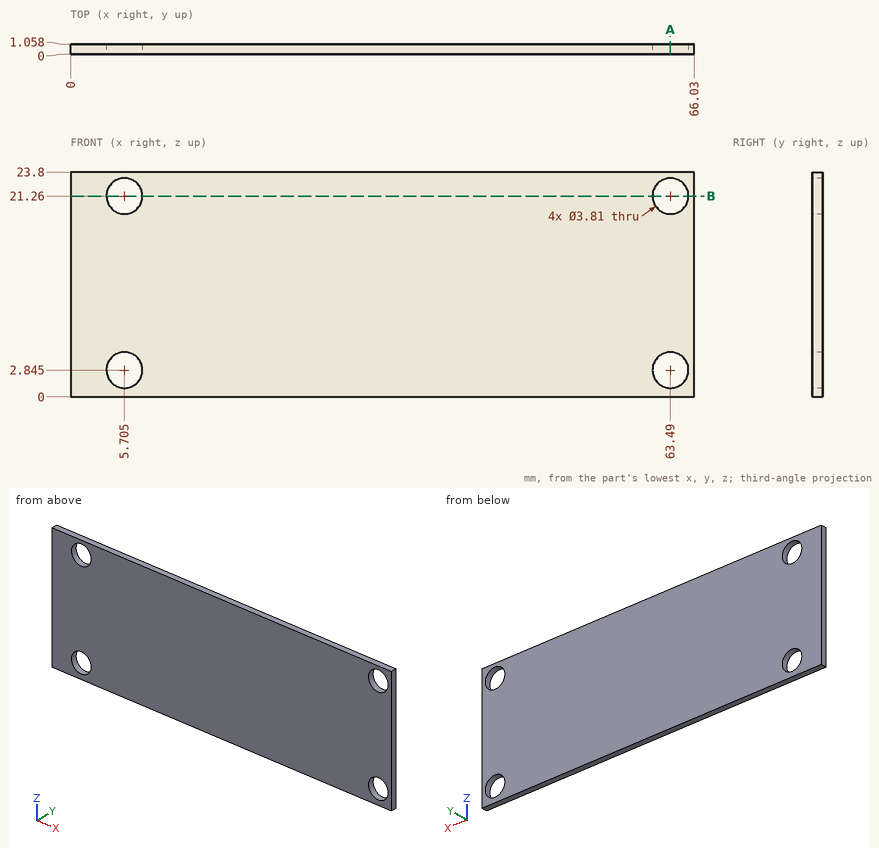
Source: three-view drawing plus pictorial views. Frame: mm from the lowest corner of the part. Coordinates: 2 decimals unless noted, no trailing zeros. Order: outer loops, then holes, each group sorted by start corner. A loop starts at its lowest first (then second) coordinate and runs counter-clockwise, first axis right, second up. Notation, with made-up numbers: M 62,33 L 68,33 A11 cw 68,49 Z; hole C 36,76.5 d1. An arc over 180 degrees is marked long. One line per question, with ' | ' between items. Start each with the question number.
Item 1: Cut plane B-B, the plane z = 21.26. Return the cut outline in (x, y) (1 decimal).
Item 2: Cut plane A-A, the plane x = 63.49. Count the separate pieces of the cut face and the enclosed holes in it, then the cut area to 3 significant figures.
Item 3: Ray query, probe 1 along X at (y, z) = (0.7, 21.26) (1 decimal); probe 2 along Z at (x, y) = (5, 0.15) (1 decimal); probe 3 along X at (y, z) = (0.8, 22.25). Return the intervals inside material, ascending. Write a range as [from, to].
Item 4: Pin query (flat end, axial travel): pin 1 Ø3.5 at (x, z) = (63.49, 2.845) entering from +Y. Return the tip coordinate at first contact, or that it passes through.
A:
1) outline: M 0,0 L 3.8,0 L 3.8,1.1 L 0,1.1 Z; M 7.6,0 L 61.6,0 L 61.6,1.1 L 7.6,1.1 Z; M 65.4,0 L 66,0 L 66,1.1 L 65.4,1.1 Z
2) separate pieces: 3 | enclosed holes: 0 | area: 17.1 mm2
3) probe 1: x = [0, 3.8], [7.6, 61.6], [65.4, 66] | probe 2: z = [0, 1.1], [4.6, 19.5], [23, 23.8] | probe 3: x = [0, 4.08], [7.33, 61.86], [65.12, 66.03]
4) pin 1: passes through
